The listing builds one solid part. Answer for the finished solid, in the listing's coordinates (mm). Face numbers are marked on the shaded views. Round coordinates to 2 decimals unless told otherwise and drop trailing zeros. Write each loop counter-clockwise with the first axis right and the second up, starting at its lowest first coordinate (ties: lowest second). Pieces come first, ordered by that corner, then holes. Notation, with made-up numbers: (75, 22) -> (108, 22) arc R14 ccw to (108, 47) -> close; hole circle Ø10 at (56, 74). An arc over 180 degrees is marked (long way). Write each question's results on one line, items separated by ' | '. Start each with the question number.
```python
from build123d import *

# Parameters (mm, degrees)
CROQUIS1_R              = 6
CROQUIS1_R_2            = 4
SALIENTE_EXTRUIR1_DEPTH = 1
CROQUIS2_R              = 7
CROQUIS2_R_2            = 6
CROQUIS2_R_3            = 4.5
CROQUIS2_R_4            = 4
SALIENTE_EXTRUIR2_DEPTH = 1.8
CROQUIS3_R              = 7
CROQUIS3_R_2            = 6
CROQUIS3_R_3            = 4.5
CROQUIS3_R_4            = 4
SALIENTE_EXTRUIR3_DEPTH = 0.2
CROQUIS4_R              = 7.99896204
CROQUIS4_R_2            = 6
CROQUIS4_R_3            = 5
CROQUIS4_R_4            = 4
SALIENTE_EXTRUIR4_DEPTH = 0.8


with BuildPart() as part:
    # Croquis1 → Saliente-Extruir1 (new body)
    with BuildSketch(Plane.XY):
        with BuildLine():
            Line((-10, -12.938825758), (-10, -33.938825758))
            ThreePointArc((-10, -33.938825758), (-5, -48.183823756), (0, -33.938825758))
            Line((0, -33.938825758), (0, -12.938825758))
            ThreePointArc((0, -12.938825758), (-5, -7.938825758), (-10, -12.938825758))
        make_face()
        with Locations((-5, -40.183823756)):
            Circle(CROQUIS1_R, mode=Mode.SUBTRACT)
        with Locations((-5, -12.938825758)):
            Circle(CROQUIS1_R_2, mode=Mode.SUBTRACT)
    extrude(amount=SALIENTE_EXTRUIR1_DEPTH)

    # Croquis2 → Saliente-Extruir2 (add)
    with BuildSketch(Plane.XY.offset(1)):
        with Locations((-5, -40.183823756)):
            Circle(CROQUIS2_R)
        with Locations((-5, -40.183823756)):
            Circle(CROQUIS2_R_2, mode=Mode.SUBTRACT)
        with Locations((-5, -12.938825758)):
            Circle(CROQUIS2_R_3)
        with Locations((-5, -12.938825758)):
            Circle(CROQUIS2_R_4, mode=Mode.SUBTRACT)
    extrude(amount=SALIENTE_EXTRUIR2_DEPTH)

    # Croquis3 → Saliente-Extruir3 (add)
    with BuildSketch(Plane(origin=(0, 0, 0), x_dir=(-1, 0, 0), z_dir=(0, 0, -1))):
        with Locations((5, -40.183823756)):
            Circle(CROQUIS3_R)
        with Locations((5, -40.183823756)):
            Circle(CROQUIS3_R_2, mode=Mode.SUBTRACT)
        with Locations((5, -12.938825758)):
            Circle(CROQUIS3_R_3)
        with Locations((5, -12.938825758)):
            Circle(CROQUIS3_R_4, mode=Mode.SUBTRACT)
    extrude(amount=SALIENTE_EXTRUIR3_DEPTH)

    # Croquis4 → Saliente-Extruir4 (add)
    with BuildSketch(Plane(origin=(0, 0, -0.2), x_dir=(-1, 0, 0), z_dir=(0, 0, -1))):
        with Locations((5, -40.183823756)):
            Circle(CROQUIS4_R)
        with Locations((5, -40.183823756)):
            Circle(CROQUIS4_R_2, mode=Mode.SUBTRACT)
        with Locations((5, -12.938825758)):
            Circle(CROQUIS4_R_3)
        with Locations((5, -12.938825758)):
            Circle(CROQUIS4_R_4, mode=Mode.SUBTRACT)
    extrude(amount=SALIENTE_EXTRUIR4_DEPTH)


solid = part.part
```
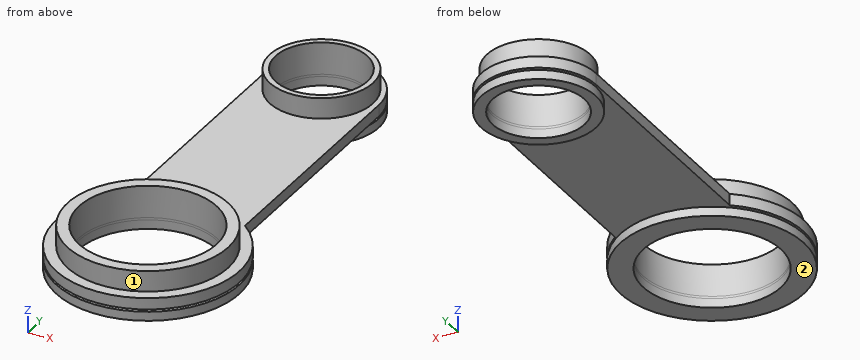
Q1. Each of these flat-tipped pins is pushed along its axis until it touches: pin 1 (1.5 mm diameter, centred on y = -38, z = 2, fed in from -X); pin 2 (1.5 mm diameter, centred on x = -9.5, z = 2, fed in from -Y); pin 3 (2 mm diameter, centred on x = -5.5, z = 0, fed in from +Y); pin 4 (5 mm diameter, centred on x = -6, y = -24, fed in from -Z). Where does it stop, or does it pass through?
Q2. The part is cut by section A-A, the plane y = -15. Write down the section's boundary in (x, z), then the cut area to 3 significant figures.
Q3. The part is cut by section C-C, the plane z = 0.35. Write down the section's boundary in (x, y).
Q4. Determine the mould class of the marked faces 1 and 2 for opening direction Y: pulls with the +Y half, pulls with the -Y half, needs draft (parallel to the pull), parting line crosses it, or undercut.
Q5. The part is cut by section B-B, the plane x = -5. State how many separate pieces and enclosed holes the cut face has, then the cut area to 3 significant figures.
Q6. Find the intervals of material crossed by line 1 (Y direction, x = -5, z = 2.2); line 2 (Y direction, x = -5, z = -0.75); line 3 (Z direction, x = -0.5, y = -34), in increasing order.
Answers follow:
1) pin 1: x = -11.85 | pin 2: y = -46.09 | pin 3: y = -7.94 | pin 4: z = 0
2) outline: (-10, 0) -> (-9, 0) -> (-9, -0.2) -> (-9.56, -0.2) -> (-9.56, -1) -> (-8.43, -1) -> (-8.43, 2.8) -> (-9, 2.8) -> (-9, 1) -> (-10, 1) -> close; (-1.57, -1) -> (-0.44, -1) -> (-0.44, -0.2) -> (-1, -0.2) -> (-1, 0) -> (0, 0) -> (0, 1) -> (-1, 1) -> (-1, 2.8) -> (-1.57, 2.8) -> close | area: 7.24 mm^2
3) outline: (-10, -33.94) arc R8 ccw (long way) to (0, -33.94) -> (0, -12.94) arc R5 ccw to (-10, -12.94) -> close; hole circle Ø12 at (-5, -40.18); hole circle Ø8 at (-5, -12.94)
4) face 1: undercut | face 2: needs draft
5) separate pieces: 3 | enclosed holes: 0 | area: 31.0 mm^2
6) line 1: -47.18 to -46.18, -34.18 to -33.18, -17.44 to -16.94, -8.94 to -8.44 | line 2: -48.18 to -46.18, -34.18 to -32.18, -17.94 to -16.94, -8.94 to -7.94 | line 3: -1 to -0.2, 0 to 1
